The drawing under review shows one solid part. Ordinate dimensions are in mm from its lowest x, y, z. A direction names the side the tool comes from. Coordinates: 2 decimals unless noted, no trailing zeros. Write each loop counter-clockwise with the first axis right and the second up, starting at its lowest first coordinate (ties: lowest second). Pieces come first, ordered by that corner, then holes. Notation, with made-up numbers: M -39.5,23 L -7.5,23 A16 cw -7.5,39 Z; hole C 37.5,84 d5. An arc over 180 degrees is marked long. Write item = value, one per line.
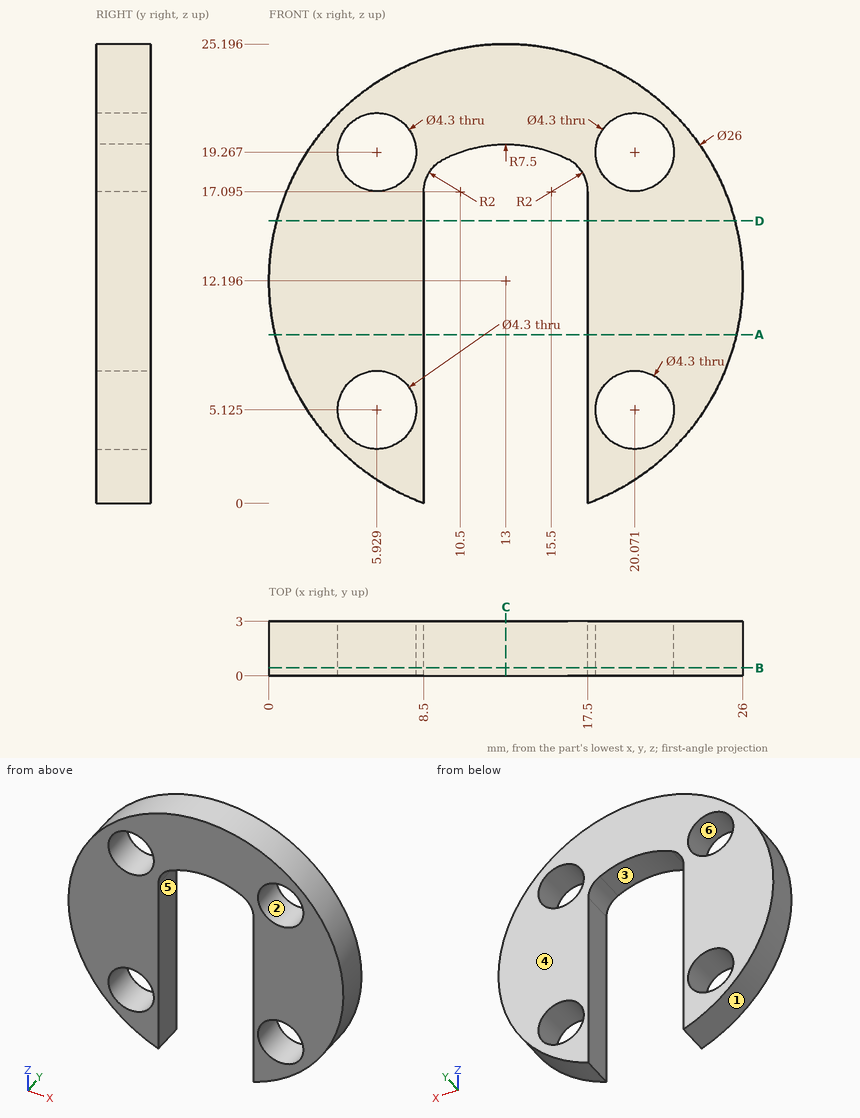
Q1. The part is to be moulded in two halves that separate along X. For the marked faces 1, 2, 3 and 4, say which applies: +X half, -X half, draft (parallel to the pull), parting line (faces both ways), or undercut.
Check result:
face_1 = parting line
face_2 = undercut
face_3 = undercut
face_4 = draft
Q2. Consider section C-C, the plane x = 13. State the section outline as (y, z) points, and give its area (3 significant figures).
Check result:
outline = M 0,19.7 L 3,19.7 L 3,25.2 L 0,25.2 Z
area = 16.5 mm²
Q3. Machinability: for the marked faces 5 and 6, which of the approach directions +Z, -Z, +X, -X, +Y, -Y give a long, thin tool a straight path to every point of the face, cutting with its end or side? Answer none if there is none.
Check result:
face_5 = -Z, +Y, -Y
face_6 = +Y, -Y
Q4. Consider section D-D, the plane z = 15.5. State the section outline as (x, y) points.
Check result:
outline = M 0.43,0 L 8.5,0 L 8.5,3 L 0.43,3 Z; M 17.5,0 L 25.57,0 L 25.57,3 L 17.5,3 Z
Q5. Wall thickness on line 1 (Z direction, x = 18.5, y = 2.8) (1 decimal); line 2 (X direction, y = 1.5, z = 6.25) (1 decimal); line 3 (X direction, y = 2.2, z = 20.25) (1 decimal): over which ranges is each line inside the solid? List them lowest first.
Check result:
line_1 = 0.4 to 3.7, 6.6 to 17.8, 20.7 to 24
line_2 = 1.4 to 4.1, 7.8 to 8.5, 17.5 to 18.2, 21.9 to 24.6
line_3 = 2.8 to 4, 7.8 to 18.2, 22 to 23.2
Q6. Consider section B-B, the plane y = 0.45. State how many separate pieces and enclosed holes the cut face has.
Check result:
separate_pieces = 1
enclosed_holes = 4
Q7. Consider section A-A, the plane z = 9.25. State the section outline as (x, y) points.
Check result:
outline = M 0.34,0 L 8.5,0 L 8.5,3 L 0.34,3 Z; M 17.5,0 L 25.66,0 L 25.66,3 L 17.5,3 Z
Q8. For P1, Ø1.5, axis at y = 1, z = 6.5, coming from the +X side; P2, Ø1, axis at y = 2, z = 14.5, coming from the -X side; P3, Ø3.5, axis at x = 5.93, z = 19.27, coming from the +Y side, all flat-tipped, find the tip position at first contact; note any pin that passes through.
Check result:
P1 = 25.02
P2 = 0.13
P3 = through
